Could you check a few things on this model? Use its own coordinates, in mm. A direction names the side the tool comes from. Coordinates: 2 decimals unless noted, no trailing zeros. Loops run counter-clockwise (first coordinate to the right, second up) from the corner with the lowest first, then second, coordinate; pieces in that order, holes last. Notation, with made-up numbers: (-19.75, -35.75) -> (-8.75, -35.75) arc R32 ccw to (-8.75, -2.75) -> close; hole circle Ø10 at (-3.75, 60.5). An arc over 180 degrees is marked (long way). One line per question, with ' | ' between items. Start each with the question number.
(1) If I drill on line 1 along X through (y, z) = (10.5, 1); line 2 along Y through (x, z) = (-19, 27); line 3 along X through (y, z) = (6, 22), over which ranges is the centre line in solid material (lowest first)?
(2) Suppose I cut it at B-B (x = -19). Please give me the cut outline in (y, z).
(3) Suppose I cut it at A-A (y = -12.5). Please give me the cut outline in (x, z).
(4) If we mould it in two halves opening along Z, with no side actions, what happens to faces 1 (the face through (-30, 25, 25)), 2 (the face through (106.763, 0.42, 11.663)), 3 (the face through (29.993, -0.66, 8.874))? For each: pulls with the +Z half, pulls with the -Z half, needs draft (parallel to the pull), parting line crosses it, or undercut.
(5) Which directions (+Z, -Z, +X, -X, +Y, -Y) give clear straight access to the entire face, cutting with the end or side of a thin tool? Please do faces 4 (the face through (-24.038, 27.535, 23.451)), 5 (the face through (69, -15, 22)), 6 (the face through (102.9, 0.4, 3)), 7 (the face through (-30, -9, 17)).
(6) Suppose I cut it at D-D (z = 22.5). Give the number of separate pieces and of enclosed holes in the cut face, plus the area to 3 significant figures.
(7) I'm going to push flat-ended pins straight in: pin 1 Ø1 at (y, z) = (-18, 24) entering from +X; pin 2 Ø18 at (x, y) = (52, -6) entering from -Z; pin 3 Ø19 at (x, z) = (-34.5, 23) entering from +Y; pin 4 Ø6 at (x, z) = (-30.5, 31.5) entering from -Y. Where does each tip first touch, or does it pass through?
(8) Suppose I cut it at C-C (y = -22.5). Please give me the cut outline in (x, z).
```python
from build123d import *
from build123d.topology import SkipClean

# Parameters (mm, degrees)
BOSS_EXTRUDE1_DEPTH                      = 45
CBORE_FOR_M10_HEX_HEAD_BOLT1_D           = 12
CBORE_FOR_M10_HEX_HEAD_BOLT1_DEPTH       = 21
CBORE_FOR_M10_HEX_HEAD_BOLT1_CBORE_D     = 24
CBORE_FOR_M10_HEX_HEAD_BOLT1_CBORE_DEPTH = 5
CBORE_FOR_M10_HEX_HEAD_BOLT1_TIP         = 3.605163714
CBORE_FOR_M10_HEX_HEAD_BOLT2_D           = 12
CBORE_FOR_M10_HEX_HEAD_BOLT2_CBORE_D     = 24
CBORE_FOR_M10_HEX_HEAD_BOLT2_CBORE_DEPTH = 5
SKETCH8_W                                = 9
SKETCH8_H                                = 60
BOSS_EXTRUDE5_DEPTH                      = 150
SKETCH11_R                               = 12
CUT_EXTRUDE3_DEPTH                       = 5
SKETCH13_R                               = 6
CUT_EXTRUDE4_DEPTH                       = 99
SKETCH14_R                               = 12
CUT_EXTRUDE5_DEPTH                       = 5
CUT_EXTRUDE6_START                       = -68
CUT_EXTRUDE6_DEPTH                       = 68
BOSS_EXTRUDE8_DEPTH                      = 60
CUT_EXTRUDE7_DEPTH                       = 68
SKETCH18_R                               = 9
CUT_EXTRUDE8_DEPTH                       = 68
CUT_EXTRUDE9_DEPTH                       = 68


with BuildPart() as part:
    # Sketch1 → Boss-Extrude1 (new body)
    with BuildSketch(Plane.XY):
        with BuildLine():
            Line((0, 30), (-60, 30))
            Line((-60, 30), (-60, 9))
            Line((-60, 9), (-12, 9))
            ThreePointArc((-12, 9), (15, 0), (-12, -9))
            Line((-12, -9), (-60, -9))
            Line((-60, -9), (-60, -30))
            Line((-60, -30), (0, -30))
            ThreePointArc((0, -30), (30, 0), (0, 30))
        make_face()
    extrude(amount=BOSS_EXTRUDE1_DEPTH)

    # CBORE for M10 Hex Head Bolt1
    with Locations(Plane(origin=(0, 30, 0), x_dir=(1, 0, 0), z_dir=(0, 1, 0))):
        with Locations((-36, -22.5)):
            CounterBoreHole(CBORE_FOR_M10_HEX_HEAD_BOLT1_D / 2, CBORE_FOR_M10_HEX_HEAD_BOLT1_CBORE_D / 2, CBORE_FOR_M10_HEX_HEAD_BOLT1_CBORE_DEPTH, depth=CBORE_FOR_M10_HEX_HEAD_BOLT1_DEPTH)
            with Locations((0, 0, -(CBORE_FOR_M10_HEX_HEAD_BOLT1_DEPTH + CBORE_FOR_M10_HEX_HEAD_BOLT1_TIP / 2))):  # 118° drill point
                Cone(0, CBORE_FOR_M10_HEX_HEAD_BOLT1_D / 2, CBORE_FOR_M10_HEX_HEAD_BOLT1_TIP, mode=Mode.SUBTRACT)

    # CBORE for M10 Hex Head Bolt2 (through all)
    with Locations(Plane(origin=(0, -30, 0), x_dir=(-1, 0, 0), z_dir=(0, -1, 0))):
        with Locations((36, -22.5)):
            CounterBoreHole(CBORE_FOR_M10_HEX_HEAD_BOLT2_D / 2, CBORE_FOR_M10_HEX_HEAD_BOLT2_CBORE_D / 2, CBORE_FOR_M10_HEX_HEAD_BOLT2_CBORE_DEPTH)

    # Sketch8 → Boss-Extrude5 (add)
    with BuildSketch(Plane.ZY.offset(60)):
        with Locations((22.5, 0)):
            Rectangle(SKETCH8_W, SKETCH8_H)
    extrude(amount=-BOSS_EXTRUDE5_DEPTH)

    # Sketch11 → Cut-Extrude3 (cut)
    with BuildSketch(Plane(origin=(0, 30, 0), x_dir=(1, 0, 0), z_dir=(0, 1, 0))):
        with Locations(Location((-36, -22.5, 0), (0, 0, 270))):
            Circle(SKETCH11_R)
    extrude(amount=-CUT_EXTRUDE3_DEPTH, mode=Mode.SUBTRACT)

    # Sketch13 → Cut-Extrude4 (cut)
    with SkipClean():  # the faces are left unmerged after this step: merging them gives an invalid solid
        with BuildSketch(Plane(origin=(0, 30, 0), x_dir=(1, 0, 0), z_dir=(0, 1, 0))):
            with Locations(Location((-36, -22.5, 0), (0, 0, 270))):
                Circle(SKETCH13_R)
        extrude(amount=-CUT_EXTRUDE4_DEPTH, mode=Mode.SUBTRACT)

    # Sketch14 → Cut-Extrude5 (cut)
    with SkipClean():  # the faces are left unmerged after this step: merging them gives an invalid solid
        with BuildSketch(Plane.XZ.offset(30)):
            with Locations(Location((-36, 22.5, 0), (0, 0, 90))):
                Circle(SKETCH14_R)
        extrude(amount=-CUT_EXTRUDE5_DEPTH, mode=Mode.SUBTRACT)

    # Sketch15 → Cut-Extrude6 (cut)
    with BuildSketch(Plane.XY.offset(27).offset(CUT_EXTRUDE6_START)):
        with BuildLine():
            Line((-12, 9), (-60, 9))
            Line((-60, 9), (-60, -9))
            Line((-60, -9), (-12, -9))
            ThreePointArc((-12, -9), (15, 0), (-12, 9))
        make_face()
    extrude(amount=CUT_EXTRUDE6_DEPTH, mode=Mode.SUBTRACT)

    # Sketch16 → Boss-Extrude8 (add)
    with BuildSketch(Plane(origin=(0, 30, 0), x_dir=(1, 0, 0), z_dir=(0, 1, 0))):
        Polygon((90, -27), (134.636969371, 13.838596515), (128.561806253, 20.478806835), (83.924836882, -20.35978968), align=None)
    extrude(amount=-BOSS_EXTRUDE8_DEPTH)

    # Sketch17 → Cut-Extrude7 (cut)
    with BuildSketch(Plane(origin=(48.380075948, 0, 52.879877188), x_dir=(-0.7378011466347597, 0, 0.6750181242192198), z_dir=(-0.6750181242192198, 0, -0.7378011466347597))):
        with BuildLine():
            Line((-51.672504688, -30), (-93.46941491, -17.594984307))
            ThreePointArc((-93.46941491, -17.594984307), (-107.672504688, 0), (-93.46941491, 17.594984307))
            Line((-93.46941491, 17.594984307), (-51.672504688, 30))
            Line((-51.672504688, 30), (-131.97504834, 46.212798572))
            Line((-131.97504834, 46.212798572), (-125.335440866, -48.202419702))
            Line((-125.335440866, -48.202419702), (-41.145218102, -48.202419702))
            Line((-41.145218102, -48.202419702), (-51.672504688, -30))
        make_face()
    extrude(amount=-CUT_EXTRUDE7_DEPTH, mode=Mode.SUBTRACT)

    # Sketch18 → Cut-Extrude8 (cut)
    with BuildSketch(Plane(origin=(48.380075948, 0, 52.879877188), x_dir=(-0.7378011466347597, 0, 0.6750181242192198), z_dir=(-0.6750181242192198, 0, -0.7378011466347597))):
        with Locations((-89.672504688, 0)):
            Circle(SKETCH18_R)
    extrude(amount=-CUT_EXTRUDE8_DEPTH, mode=Mode.SUBTRACT)

    # Sketch19 → Cut-Extrude9 (cut)
    with BuildSketch(Plane(origin=(0, 0, 18), x_dir=(-1, 0, 0), z_dir=(0, 0, -1))):
        with BuildLine():
            Line((-69, 0), (-69, -30))
            Line((-69, -30), (-51, -30))
            Line((-51, -30), (-51, 0))
            ThreePointArc((-51, 0), (-60, 9), (-69, 0))
        make_face()
    extrude(amount=-CUT_EXTRUDE9_DEPTH, mode=Mode.SUBTRACT)


solid = part.part
```
Checks:
1) line 1: x = -60 to -10.71, 10.71 to 28.1, 105.09 to 118.42 | line 2: y = -30 to -9, 9 to 30 | line 3: x = 13.75 to 53.29, 66.71 to 95.47
2) outline: (-30, 0) -> (-9, 0) -> (-9, 45) -> (-30, 45) -> close; (9, 0) -> (30, 0) -> (30, 45) -> (9, 45) -> close
3) outline: (-60, 0) -> (-8.29, 0) -> (-8.29, 45) -> (-60, 45) -> close; (8.29, 0) -> (27.27, 0) -> (27.27, 18) -> (51, 18) -> (51, 27) -> (27.27, 27) -> (27.27, 45) -> (8.29, 45) -> close; (69, 18) -> (86.5, 18) -> (124.1, -16.39) -> (130.17, -9.75) -> (90, 27) -> (69, 27) -> close; hole circle Ø12 at (-36, 22.5)
4) face 1: undercut | face 2: pulls with the +Z half | face 3: needs draft
5) face 4: +Y | face 5: +Z, -Z, -Y | face 6: -Z, +Y, -Y | face 7: +Z, -Z, -X
6) separate pieces: 3 | enclosed holes: 0 | area: 6,470 mm^2
7) pin 1: stops at x = 93.83 | pin 2: stops at z = 18 | pin 3: stops at y = 25 | pin 4: stops at y = -30
8) outline: (-60, 0) -> (19.84, 0) -> (19.84, 18) -> (51, 18) -> (51, 27) -> (19.84, 27) -> (19.84, 45) -> (-60, 45) -> close; (69, 18) -> (86.5, 18) -> (105.15, 0.94) -> (111.22, 7.58) -> (90, 27) -> (69, 27) -> close; hole circle Ø12 at (-36, 22.5)
